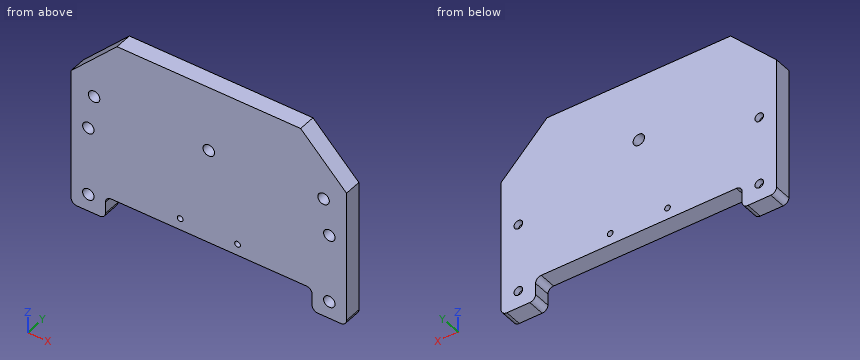
from build123d import *

# Parameters (mm, degrees)
F1_DEPTH       = 19.05
F2_R           = 6.35
F3_SIZE2       = 50.8
F3_SIZE        = 50.8
F4_R           = 6.35
F4_R_2         = 3.175
F5_DEPTH       = 25.4
F6_D           = 12.7
F6_DEPTH       = 12.7
F6_TIP         = 3.8154649308
F7_D           = 9.525
F7_DEPTH       = 25.4
F7_CBORE_D     = 12.7
F7_CBORE_DEPTH = 12.7
F7_TIP         = 2.8615986981


with BuildPart() as f1:
    # F0 (on Front) → F1 (new body)
    with BuildSketch(Plane.XZ):
        Polygon((-61.5315027535, 184.1499997646), (-61.5315027535, -19.0500002354), (-23.4315027535, -19.0500002354), (-23.4315027535, 6.3499997646), (205.1684972465, 6.3499997646), (205.1684972465, -19.0500002354), (243.2684972465, -19.0500002354), (243.2684972465, 184.1499997646), align=None)
    extrude(amount=F1_DEPTH)

    # F2
    f2_edges = [f1.edges().sort_by_distance(p)[0] for p in [
        (-23.431503, -9.525, 6.35),
        (-61.531503, -9.525, -19.05),
        (243.268497, -9.525, -19.05),
        (205.168497, -9.525, -19.05),
        (205.168497, -9.525, 6.35),
        (-23.431503, -9.525, -19.05),
    ]]
    fillet(f2_edges, radius=F2_R)

    # F3
    f3_edges = [f1.edges().sort_by_distance(p)[0] for p in [
        (243.268497, -9.525, 184.15),
        (-61.531503, -9.525, 184.15),
    ]]
    chamfer(f3_edges, length=F3_SIZE, length2=F3_SIZE2)

    # F4 (on face) → F5 (cut)
    with BuildSketch(Plane.XZ.offset(19.05)):
        with Locations((90.8684972465, 111.9631997646)):
            Circle(F4_R)
        with Locations((59.1184972465, 19.0499997646)):
            Circle(F4_R_2)
        with Locations((122.6184972465, 19.0499997646)):
            Circle(F4_R_2)
    extrude(amount=-F5_DEPTH, mode=Mode.SUBTRACT)

    # F6
    with Locations(Plane.XZ.offset(19.05)):
        with Locations((-36.1315027535, 115.1381997646), (217.8684972465, 115.1381997646)):
            Hole(F6_D / 2, depth=F6_DEPTH)
            with Locations((0, 0, -(F6_DEPTH + F6_TIP / 2))):  # 118° drill point
                Cone(0, F6_D / 2, F6_TIP, mode=Mode.SUBTRACT)

    # F7
    with Locations(Plane.XZ.offset(19.05)):
        with Locations((-42.4815027535, 76.1999997646), (-42.4815027535, -2.354e-07), (224.2184972465, -2.354e-07), (224.2184972465, 76.1999997646)):
            CounterBoreHole(F7_D / 2, F7_CBORE_D / 2, F7_CBORE_DEPTH, depth=F7_DEPTH)
            with Locations((0, 0, -(F7_DEPTH + F7_TIP / 2))):  # 118° drill point
                Cone(0, F7_D / 2, F7_TIP, mode=Mode.SUBTRACT)


solid = f1.part
Geometry: final body of the model. Coordinates: model frame, mm. Give positions to 0.01 mm unless a question says otherwise; leave off trailing zeros. Loops run counter-clockwise (first coordinate to the right, second up) from the corner with the lowest first, then second, coordinate; pieces in that order, holes last. Notation, with made-up numbers: (-31.5, -32) - (3.5, -32) arc R33 ccw to (3.5, 3) - close; hole circle Ø10 at (-5.5, 52.25). An arc over 180 degrees is marked (long way). One line per question, with ' | ' between items. Start each with the question number.
(1) Section query B-B on y = -14.25. Count the separate pieces of the cut face and the enclosed holes in it, then the cut area to 3 significant figures.
(2) Section query C-C on z = 19.05. Return loops of the section in (x, y), then the cut area to 3 significant figures.
(3) Section query D-D on x = 9. Return loops of the section in (y, z).
(4) Ray query, line 1 (X direction, y = -1.5, z = 76.2); line 2 (X direction, y = -15.5, z = 76.2); line 3 (X direction, y = -5, z = -2). Return the intervals inside material, ascending. Write a range as from..to.
(5) Contact query for flat-ended pins moving along their axis: pin 1 (10 mm diameter, centred on x = -42.48, z = 0, fed in from -Y); pin 2 (4 mm diameter, centred on x = 56, y = -8, fed in from -Z); pin 3 (5 mm diameter, centred on x = -19.5, y = -8.5, fed in from +Z); pin 4 (8.5 mm diameter, centred on x = -42.48, z = 0, fed in from -Y). Output: stop coordinate, or through.
(6) Section query A-A on z = 76.2. Return loops of the section in (x, y), then the cut area to 3 significant figures.
The answers:
1) separate pieces: 1 | enclosed holes: 9 | area: 52,600 mm2
2) outline: (-61.53, -19.05) - (55.94, -19.05) - (55.94, 0) - (-61.53, 0) - close; (62.29, -19.05) - (119.44, -19.05) - (119.44, 0) - (62.29, 0) - close; (125.79, -19.05) - (243.27, -19.05) - (243.27, 0) - (125.79, 0) - close | area: 5,560 mm2
3) outline: (-19.05, 6.35) - (0, 6.35) - (0, 184.15) - (-19.05, 184.15) - close
4) line 1: -61.53..-47.24, -37.72..219.46, 228.98..243.27 | line 2: -61.53..-48.83, -36.13..217.87, 230.57..243.27 | line 3: -61.53..-46.8, -38.16..-23.43, 205.17..219.9, 228.54..243.27
5) pin 1: y = -6.35 | pin 2: z = 6.35 | pin 3: z = 177.88 | pin 4: through
6) outline: (-61.53, -19.05) - (-48.83, -19.05) - (-48.83, -6.35) - (-47.24, -6.35) - (-47.24, 0) - (-61.53, 0) - close; (-37.72, -6.35) - (-36.13, -6.35) - (-36.13, -19.05) - (217.87, -19.05) - (217.87, -6.35) - (219.46, -6.35) - (219.46, 0) - (-37.72, 0) - close; (228.98, -6.35) - (230.57, -6.35) - (230.57, -19.05) - (243.27, -19.05) - (243.27, 0) - (228.98, 0) - close | area: 5,360 mm2
